Verification items for the finished model (mm, model axes). Face numbers are marked on the shaded views. Round coordinates to 2 decimals unless told otherwise and drop trailing zeros. Order: outer loops, then holes, each group sorted by start corner. A loop starts at its lowest first (then second) coordinate and runs counter-clockwise, first axis right, second up. Notation, with made-up numbers: (49, 51.5) -> (62, 51.5) arc R21 cw to (62, 56.5) -> close; hole circle Ø11 at (-38.75, 76). An arc over 180 degrees is marked (long way). Return JSON: item names as keys, results as strings. Group by question number.
Item 1: Sectioned sample at C-C on x = -1. Record the cut outline in (y, z) (3 decimals), plus the area to 3 significant figures.
Item 2: Sectioned sample at A-A on z = 0. Record the cut outline in (x, y).
Item 3: Scan lines: probe 1 along Y at (x, z) = (9.5, 11); probe 2 along Y at (x, z) = (37, 13); probe 3 along X at (y, z) = (4.5, -11). Record each from-to range of solid material in increasing order. Write a range as from..to.
Item 4: Sectioned sample at D-D on x = 16.5. Record the cut outline in (y, z) (3 decimals), plus the area to 3 significant figures.
Item 5: Sectioned sample at B-B on y = 12.5. Give the number of separate pieces and of enclosed holes in the cut face, plus the area to 3 significant figures.
Item 6: Draft check along Z on the marked faces 1, 2, 3 and 4. Enter one of: pulls with the +Z half, pulls with the -Z half, needs draft (parallel to the pull), parting line crosses it, or undercut.
Item 7: Depth check by flat-ended pin: pin 1 Ø1.5 at (x, y) = (48, 28) entering from -Z; pin 2 Ø9 at (x, y) = (-8.45, 15.88) entering from +Z; pin 3 Ø1.5 at (x, y) = (-12.5, 16) entering from +Z. Enter the tip coordinate at first touch or a pass-through.
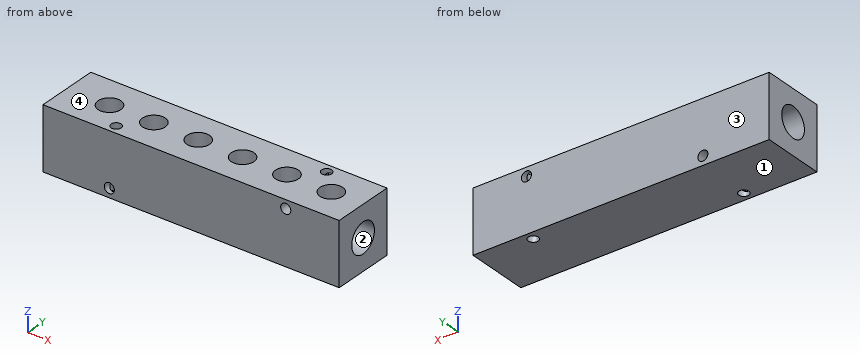
```python
from build123d import *

# Parameters (mm, degrees)
F0_W     = 149.225
F0_H     = 31.496
F1_DEPTH = 31.75
F2_R     = 5.754688
F3_DEPTH = 15.875
F4_R     = 7.540625
F5_DEPTH = 149.226
F6_R     = 2.54
F7_DEPTH = 31.751
F8_R     = 2.54
F9_DEPTH = 31.497


with BuildPart() as f1:
    # F0 (on Front) → F1 (new body)
    with BuildSketch(Plane.XZ):
        Rectangle(F0_W, F0_H)
    extrude(amount=-F1_DEPTH)

    # F2 (on Top) → F3 (cut)
    with BuildSketch(Plane.XY):
        with Locations((-53.1495, 15.875)):
            Circle(F2_R)
        with Locations((-30.7975, 15.875)):
            Circle(F2_R)
        with Locations((-8.4455, 15.875)):
            Circle(F2_R)
        with Locations((13.9065, 15.875)):
            Circle(F2_R)
        with Locations((36.2585, 15.875)):
            Circle(F2_R)
        with Locations((58.6105, 15.875)):
            Circle(F2_R)
    extrude(amount=F3_DEPTH, mode=Mode.SUBTRACT)

    # F4 (on face) → F5 (cut, through all)
    with BuildSketch(Plane.YZ.offset(74.6125)):
        with Locations((15.875, 0)):
            Circle(F4_R)
    extrude(amount=-F5_DEPTH, mode=Mode.SUBTRACT)

    # F6 (on face) → F7 (cut, through all)
    with BuildSketch(Plane.XZ):
        with Locations((-41.2115, -11.176)):
            Circle(F6_R)
        with Locations((47.6885, 11.43)):
            Circle(F6_R)
    extrude(amount=-F7_DEPTH, mode=Mode.SUBTRACT)

    # F8 (on face) → F9 (cut, through all)
    with BuildSketch(Plane.XY.offset(15.748)):
        with Locations((47.6885, 27.178)):
            Circle(F8_R)
        with Locations((-41.2115, 4.572)):
            Circle(F8_R)
    extrude(amount=-F9_DEPTH, mode=Mode.SUBTRACT)


solid = f1.part
```
Recorded:
{
 "1": {"outline": "(0, -15.748) -> (31.75, -15.748) -> (31.75, 15.748) -> (0, 15.748) -> close; hole circle Ø15.081 at (15.875, 0)", "area": "821 mm²"},
 "2": {"outline": "(-74.61, 0) -> (74.61, 0) -> (74.61, 8.33) -> (-74.61, 8.33) -> close; (-74.61, 23.42) -> (74.61, 23.42) -> (74.61, 31.75) -> (-74.61, 31.75) -> close; hole circle Ø5.08 at (-41.21, 4.57); hole circle Ø5.08 at (47.69, 27.18)"},
 "3": {"probe 1": "0..12.17, 19.58..31.75", "probe 2": "0..10.17, 21.58..31.75", "probe 3": "-74.61..-43.75, -38.67..74.61"},
 "4": {"outline": "(0, -15.748) -> (31.75, -15.748) -> (31.75, 15.748) -> (21.012, 15.748) -> (21.012, 5.52) arc R7.541 cw (long way) to (10.738, 5.52) -> (10.738, 15.748) -> (0, 15.748) -> close", "area": "731 mm²"},
 "5": {"separate pieces": "8", "enclosed holes": "2", "area": "2,140 mm²"},
 "6": {"face 1": "pulls with the -Z half", "face 2": "undercut", "face 3": "needs draft", "face 4": "pulls with the +Z half"},
 "7": {"pin 1": "through", "pin 2": "z = -6.05", "pin 3": "z = -7.49"}
}
